Input: part model. Units: mm. Frame: model coordinates. A direction names the side the tool comes from. Round coordinates to 2 decimals unless told otherwise and drop trailing zeros. Loops run counter-clockwise (first coordinate to the right, second up) from the corner with the lowest first, then second, coordinate; pieces in that order, holes last. Notation, with made-up numbers: M 12,59.25 L 49,59.25 A17 ccw 49,86.25 Z; hole C 52.25,28 d3. An arc over 180 degrees is marked long. Return JSON: item names as keys, results as strings. Group by question number.
1) Section A-A (z = 54). Output: boundary loops of the cut face in (x, y).
2) Section C-C (x = -6). Output: boundary loops of the cut face in (y, z).
3) Contact query for flat-ended pins moving along their axis: P1, Ø3, axis at x = 0.5, y = -0.5, coming from the -Z side; P2, Ø4, axis at x = -3, y = 2, coming from the +Z side; P3, Ø4, axis at y = 1, z = 50.5, coming from the -X side. Output: stop coordinate, or through.
4) Mould query, pull axis X, two halves, no side actions, for faces 1 (the face through (0, 0, 62.04)), 2 (the face through (0, 0, 82.04)), 3 (the face through (-4, 0, 58)), 4 (the face through (-0.06, 3.05, 41.23)). Classes: +X half, -X half, draft (parallel to the pull), parting line (faces both ways), or undercut.
5) Access query for faces 5 (the face through (-1, 7.75, 18)), 6 (the face through (1, 10, 0)), 7 (the face through (-5.1, 10, 7)). Directions: +Z, -Z, +X, -X, +Y, -Y. A direction counts if a zero-diameter tool reaches every point of the face in a straight line with its end or side. Return the directions, or none.
6) Section B-B (x = 0). Count the separate pieces of the cut face and the enclosed holes in it, plus the area to 3 significant figures.
7) Material intervals for line 1 (Y direction, x = -3.75, z = 55); line 2 (Y direction, x = -2, z = 17); line 3 (X direction, y = 0.75, z = 61), sorted ascending. Write a range as from..to.
from build123d import *

# Parameters (mm, degrees)
SKETCH1_W                = 8
SKETCH1_H                = 3.5
BASE_DEPTH               = 50
SKETCH3_W                = 8
SKETCH3_H                = 3.5
SEGMENT1_DEPTH           = 50
BOSS_EXTRUDE7_DEPTH      = 3.5
BOSS_EXTRUDE9_DEPTH      = 11
CUT_EXTRUDE10_DEPTH      = 101.920760996
CUT_EXTRUDE10_DEPTH_BACK = 101.920760996
CUT_EXTRUDE9_DEPTH       = 102.52124162
CUT_EXTRUDE9_DEPTH_BACK  = 102.52124162
BOSS_EXTRUDE13_DEPTH     = 3.5
CUT_EXTRUDE12_DEPTH      = 10
CUT_EXTRUDE13_DEPTH      = 105.885652022
LPATTERN3_COUNT          = 5
LPATTERN3_PITCH          = 5
BOSS_EXTRUDE14_DEPTH     = 5
FILLET5_R                = 1


with BuildPart() as part:
    # Sketch1 → Base (new body)
    with BuildSketch(Plane.XY):
        Rectangle(SKETCH1_W, SKETCH1_H)
    extrude(amount=BASE_DEPTH)

    # Sketch3 → Segment1 (add)
    with BuildSketch(Plane(origin=(0, 0, 50), x_dir=(-1, 0, 0), z_dir=(0, 0, 1))):
        Rectangle(SKETCH3_W, SKETCH3_H)
    extrude(amount=SEGMENT1_DEPTH)

    # Sketch12 → Boss-Extrude7 (add)
    with BuildSketch(Plane(origin=(0, 1.75, 0), x_dir=(1, 0, 0), z_dir=(0, 1, 0))):
        Polygon((-4, 0), (-8, 0), (-8, -7), (-4, -21.92820323), align=None)
    extrude(amount=-BOSS_EXTRUDE7_DEPTH)

    # Sketch14 → Boss-Extrude9 (add)
    with BuildSketch(Plane(origin=(0, 1.75, 0), x_dir=(1, 0, 0), z_dir=(0, 1, 0))):
        with BuildLine():
            Line((4, -50), (4, -2))
            Line((4, -2), (0, 0))
            Line((0, 0), (-2, 0))
            ThreePointArc((-2, 0), (-6.242640687, -1.757359313), (-8, -6))
            Line((-8, -6), (-8, -8))
            Line((-8, -8), (-4, -21.92820323))
            Line((-4, -21.92820323), (-4, -50))
            Line((-4, -50), (4, -50))
        make_face()
        with BuildLine():
            ThreePointArc((-5.1, -6), (-2, -2.9), (1.1, -6))
            Line((1.1, -6), (1.1, -8))
            ThreePointArc((1.1, -8), (-2, -11.1), (-5.1, -8))
            Line((-5.1, -8), (-5.1, -6))
        make_face(mode=Mode.SUBTRACT)
    extrude(amount=BOSS_EXTRUDE9_DEPTH)

    # Sketch14<2> → Cut-Extrude10 (cut, two sides: drawn at the far end of the back side and taken through both)
    with BuildSketch(Plane(origin=(0, 1.75, 0), x_dir=(1, 0, 0), z_dir=(0, 1, 0)).offset(-CUT_EXTRUDE10_DEPTH_BACK)):
        Polygon((0, 0), (4, -2), (4, 0), align=None)
        with BuildLine():
            ThreePointArc((-8, -6), (-6.242640687, -1.757359313), (-2, 0))
            Line((-2, 0), (-8, 0))
            Line((-8, 0), (-8, -6))
        make_face()
        with BuildLine():
            ThreePointArc((1.1, -6), (-2, -2.9), (-5.1, -6))
            Line((-5.1, -6), (-5.1, -8))
            ThreePointArc((-5.1, -8), (-2, -11.1), (1.1, -8))
            Line((1.1, -8), (1.1, -6))
        make_face()
    extrude(amount=CUT_EXTRUDE10_DEPTH + CUT_EXTRUDE10_DEPTH_BACK, mode=Mode.SUBTRACT)

    # Sketch16 → Cut-Extrude9 (cut, two sides: drawn at the far end of the back side and taken through both)
    with BuildSketch(Plane(origin=(4, 0, 0), x_dir=(0, 0, -1), z_dir=(1, 0, 0)).offset(-CUT_EXTRUDE9_DEPTH_BACK)):
        with BuildLine():
            Line((-50, 12.75), (-50, 1.75))
            Line((-50, 1.75), (-49.484827557, 1.75))
            ThreePointArc((-49.484827557, 1.75), (-47.984827557, 2.151923789), (-46.886751346, 3.25))
            Line((-46.886751346, 3.25), (-42.267949192, 11.25))
            ThreePointArc((-42.267949192, 11.25), (-41.169872981, 12.348076211), (-39.669872981, 12.75))
            Line((-39.669872981, 12.75), (-50, 12.75))
        make_face()
        with BuildLine():
            ThreePointArc((-43.133974596, -0.25), (-44.232050808, -1.348076211), (-45.732050808, -1.75))
            Line((-45.732050808, -1.75), (0, -1.75))
            Line((0, -1.75), (0, 7.75))
            Line((0, 7.75), (-36.783121635, 7.75))
            ThreePointArc((-36.783121635, 7.75), (-38.283121635, 7.348076211), (-39.381197846, 6.25))
            Line((-39.381197846, 6.25), (-43.133974596, -0.25))
        make_face()
    extrude(amount=CUT_EXTRUDE9_DEPTH + CUT_EXTRUDE9_DEPTH_BACK, mode=Mode.SUBTRACT)

    # Sketch22 → Boss-Extrude13 (add)
    with BuildSketch(Plane(origin=(0, 1.75, 0), x_dir=(1, 0, 0), z_dir=(0, 1, 0))):
        with BuildLine():
            Line((-4, -100), (4, -100))
            ThreePointArc((4, -100), (0, -104), (-4, -100))
        make_face()
    extrude(amount=-BOSS_EXTRUDE13_DEPTH)

    # Sketch23 → Cut-Extrude12 (cut)
    with BuildSketch(Plane.ZY.offset(4)):
        with BuildLine():
            Line((49.698901561, -0.75), (50.270753554, -0.75))
            ThreePointArc((50.270753554, -0.75), (50.557541772, -0.840423978), (50.740599864, -1.078989928))
            Line((50.740599864, -1.078989928), (50.984827557, -1.75))
            Line((50.984827557, -1.75), (48.984827557, -1.75))
            Line((48.984827557, -1.75), (49.22905525, -1.078989928))
            ThreePointArc((49.22905525, -1.078989928), (49.412113342, -0.840423978), (49.698901561, -0.75))
        make_face()
    extrude(amount=-CUT_EXTRUDE12_DEPTH, mode=Mode.SUBTRACT)

    # Sketch24 → Cut-Extrude13 (cut, symmetric)
    with BuildSketch(Plane(origin=(0, 1.75, 0), x_dir=(1, 0, 0), z_dir=(0, 1, 0))):
        with BuildLine():
            Line((1.322611054, -58.96), (-1.322611054, -58.96))
            ThreePointArc((-1.322611054, -58.96), (-2.03, -60.5), (-1.322611054, -62.04))
            Line((-1.322611054, -62.04), (1.322611054, -62.04))
            ThreePointArc((1.322611054, -62.04), (1.844695156, -61.347348677), (2.03, -60.5))
            ThreePointArc((2.03, -60.5), (1.844695156, -59.652651323), (1.322611054, -58.96))
        make_face()
    cut_extrude13 = extrude(amount=CUT_EXTRUDE13_DEPTH, both=True, mode=Mode.SUBTRACT)

    # LPattern3: Cut-Extrude13 ×5
    with Locations(*[(0, 0, i * LPATTERN3_PITCH) for i in range(1, LPATTERN3_COUNT)]):
        add(cut_extrude13, mode=Mode.SUBTRACT)

    # Sketch25 → Boss-Extrude14 (add)
    with BuildSketch(Plane(origin=(0, 12.75, 0), x_dir=(1, 0, 0), z_dir=(0, 1, 0))):
        Polygon((4, -2), (4, 0), (0, 0), align=None)
    extrude(amount=-BOSS_EXTRUDE14_DEPTH)

    # Fillet5
    fillet5_edges = [part.edges().sort_by_distance(p)[0] for p in [
        (0, -1.75, 50.984827557),
        (0, -1.75, 48.984827557),
    ]]
    fillet(fillet5_edges, radius=FILLET5_R)


solid = part.part
Returned:
{
 "1": {"outline": "M -4,-1.75 L 4,-1.75 L 4,1.75 L -4,1.75 Z"},
 "2": {"outline": "M 7.75,1.53 L 12.75,1.53 L 12.75,14.96 L 7.75,14.96 Z"},
 "3": {"P1": "stops at z = 42.41", "P2": "stops at z = 103.87", "P3": "stops at x = -4"},
 "4": {"face 1": "undercut", "face 2": "undercut", "face 3": "-X half", "face 4": "draft"},
 "5": {"face 5": "-Z, +X, -X, -Y", "face 6": "-Z, +X, -X, +Y, -Y", "face 7": "+Y, -Y"},
 "6": {"separate pieces": "7", "enclosed holes": "0", "area": "373 mm^2"},
 "7": {"line 1": "y = -1.75..1.75", "line 2": "y = 7.75..12.75", "line 3": "x = -4..-1.97, 1.97..4"}
}
